from build123d import *

# Parameters (mm, degrees)
ESQUISSE1_W          = 112
ESQUISSE1_H          = 112
BOSS_EXTRU_1_DEPTH   = 3.175
D_GAGEMENT_M41_D     = 3.7
D_GAGEMENT_M41_DEPTH = 3.175
D_GAGEMENT_M41_TIP   = 1.111592145
D_GAGEMENT_M32_D     = 2.6
D_GAGEMENT_M32_DEPTH = 3.175
D_GAGEMENT_M32_TIP   = 0.781118805


with BuildPart() as part:
    # Esquisse1 → Boss.-Extru.1 (new body)
    with BuildSketch(Plane(origin=(0, 0, 0), x_dir=(1, 0, 0), z_dir=(0, 1, 0))):
        Rectangle(ESQUISSE1_W, ESQUISSE1_H)
    extrude(amount=BOSS_EXTRU_1_DEPTH)

    # Dégagement M41
    with Locations(Plane(origin=(0, 3.175, 0), x_dir=(1, 0, 0), z_dir=(0, 1, 0))):
        with Locations((-36, -47), (36, -47)):
            Hole(D_GAGEMENT_M41_D / 2, depth=D_GAGEMENT_M41_DEPTH)
            with Locations((0, 0, -(D_GAGEMENT_M41_DEPTH + D_GAGEMENT_M41_TIP / 2))):  # 118° drill point
                Cone(0, D_GAGEMENT_M41_D / 2, D_GAGEMENT_M41_TIP, mode=Mode.SUBTRACT)

    # Dégagement M32
    with Locations(Plane(origin=(0, 3.175, 0), x_dir=(1, 0, 0), z_dir=(0, 1, 0))):
        with Locations((42, 8), (-42, 8)):
            Hole(D_GAGEMENT_M32_D / 2, depth=D_GAGEMENT_M32_DEPTH)
            with Locations((0, 0, -(D_GAGEMENT_M32_DEPTH + D_GAGEMENT_M32_TIP / 2))):  # 118° drill point
                Cone(0, D_GAGEMENT_M32_D / 2, D_GAGEMENT_M32_TIP, mode=Mode.SUBTRACT)


solid = part.part
Model file for the job. Use its own axes, mm. Give positions to 0.01 mm unless a question says otherwise; leave off trailing zeros. Write each loop counter-clockwise with the first axis right and the second up, starting at its lowest first coordinate (ties: lowest second). Pieces come first, ordered by that corner, then holes. Notation, with made-up numbers: M 18,10.5 L 63,10.5 A16 cw 63,41.5 Z; hole C 30.25,-31 d7. An arc over 180 degrees is marked long. One line per item, written item: value. Start each with the question number.
Q1. Saw through at A-A, the plane z = -8. Write the cut outline in (x, y) (3 decimals), plus the area to 3 significant figures.
Q2. Drop a flat-ended pin along its axis: pin 1 Ø2 at (x, z) = (36, 47) entering from -Y. Give the stop position or say it passes through.
Q3. Saw through at B-B, the plane x = -36. Write the cut outline in (y, z) (3 decimals).
Q4. Saw through at C-C, the plane z = 47. Write the cut outline in (x, y) (3 decimals), plus the area to 3 significant figures.
Q5. Two-plate mould, pull along X, no slides. Class faces 1 (the flat face through (-1, 3.175, -1)), 2 (the cylindrical face through (43.3, 1.57, -8.06)), 3 (the flat face through (-56, 2, 1)): +X half, -X half, draft (parallel to the pull), parting line (faces both ways), or undercut.
Q6. Probe probe 1 along X at (y, z) = (2.35, -8); probe 2 along X at (y, z) = (0.8, 47); probe 3 along Z at (x, y) = (42, 2.95). List the from-to ranges inside material, lowest first. Write a range as [from, to].
Output values:
1. outline: M -56,0 L -43.3,0 L -43.3,3.175 L -56,3.175 Z; M -40.7,0 L 40.7,0 L 40.7,3.175 L -40.7,3.175 Z; M 43.3,0 L 56,0 L 56,3.175 L 43.3,3.175 Z
1. area: 339 mm²
2. pin 1: passes through
3. outline: M 0,-56 L 3.175,-56 L 3.175,45.15 L 0,45.15 Z; M 0,48.85 L 3.175,48.85 L 3.175,56 L 0,56 Z
4. outline: M -56,0 L -37.85,0 L -37.85,3.175 L -56,3.175 Z; M -34.15,0 L 34.15,0 L 34.15,3.175 L -34.15,3.175 Z; M 37.85,0 L 56,0 L 56,3.175 L 37.85,3.175 Z
4. area: 332 mm²
5. face 1: draft
5. face 2: undercut
5. face 3: -X half
6. probe 1: x = [-56, -43.3], [-40.7, 40.7], [43.3, 56]
6. probe 2: x = [-56, -37.85], [-34.15, 34.15], [37.85, 56]
6. probe 3: z = [-56, -9.3], [-6.7, 56]
